Geometry check sheet. Reference: drawing and pictorial views, mm from the part's lowest x, y, z. Give positions to 0.01 mm unless a question says otherwise; leave off trailing zeros. Order: outer loops, then holes, each group sorted by start corner. A loop starts at its lowest first (then second) coordinate and runs counter-clockwise, first axis right, second up.
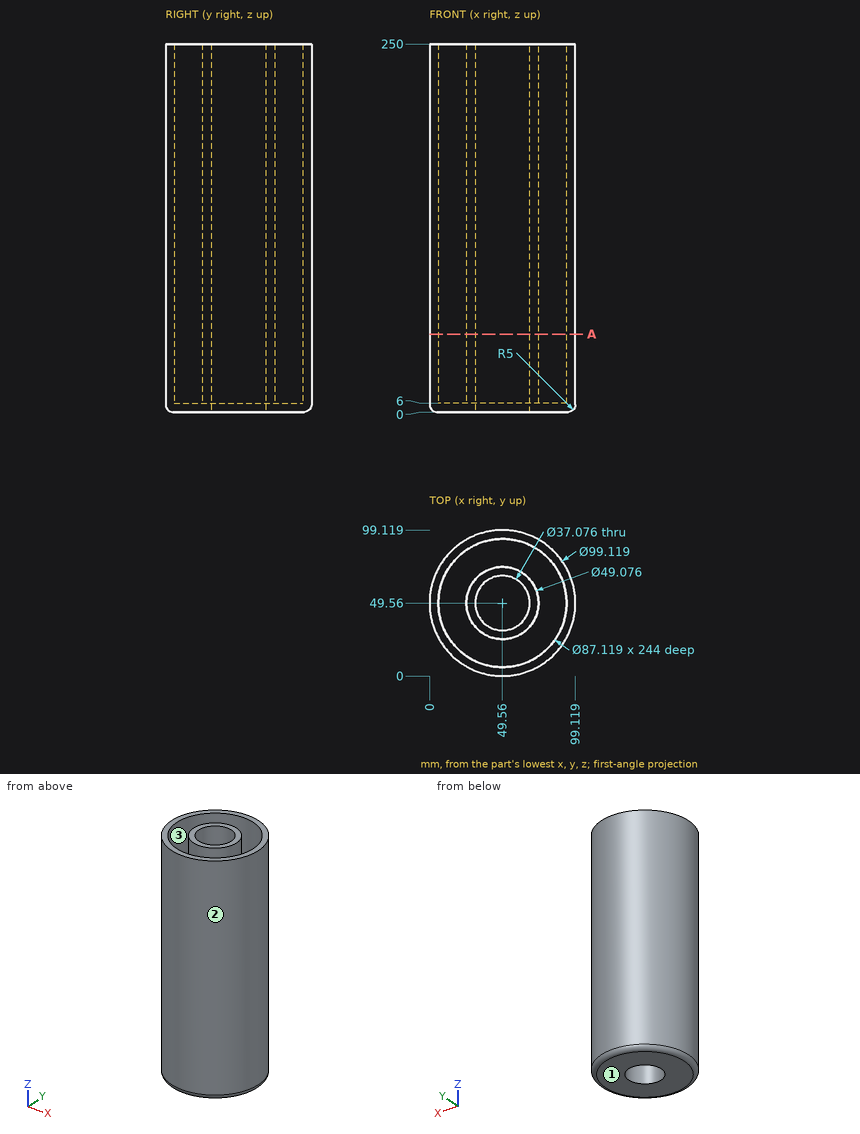
(1) Go/stop test with flat-tipped pins: P1, Ø6, axis at x = 26, z = 58, coming from the -Y side (1 decimal); P2, Ø5, axis at x = 71.5, y = 22, coming from the +Z side; P3, Ø5, axis at y = 12.5, z = 189.5, coming from the -X side. Record where each tip stops, or that it passes through.
(2) Sectioned sample at A-A (z = 53). Enter the section's corners in (x, y), plus the area to 3 significant figures.
(3) Release check for a two-part mould opening along Y. For the marked faces 1, 2 and 3 record: released by +Y, released by -Y, zero draft, split by the parting line, or undercut.
(4) Thickness scan on L1, parallel to Y at x = 48, z = 13 (1 decimal); L2, parallel to X at y = 52, z = 78.5; L3, parallel to X at y = 60.5, z = 30 (1 decimal). Record the ranges inside material, lowest first.
Values follow:
1. P1: stops at y = 4.5
1. P2: stops at z = 6
1. P3: stops at x = 14.04
2. outline: circle Ø99.12 at (49.56, 49.56); circle Ø49.08 at (49.56, 49.56); hole circle Ø87.12 at (49.56, 49.56); hole circle Ø37.08 at (49.56, 49.56)
2. area: 2,570 mm2
3. face 1: zero draft
3. face 2: split by the parting line
3. face 3: undercut
4. L1: y = 0 to 6, 25.1 to 31.1, 68 to 74, 93.1 to 99.1
4. L2: x = 0.06 to 6.07, 25.14 to 31.18, 67.94 to 73.98, 93.05 to 99.06
4. L3: x = 1.2 to 7.4, 27.6 to 34.6, 64.5 to 71.5, 91.7 to 97.9
